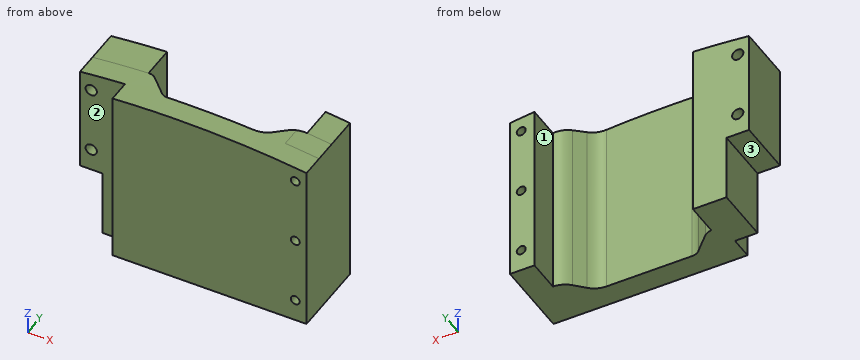
Autodesk Inventor part; units mm, degrees
ref_plane "YZ Plane" through (0, 0, 0) normal (1, 0, 0) x (0, 1, 0)
ref_plane "XZ Plane" through (0, 0, 0) normal (0, 1, 0) x (-1, 0, 0)
ref_plane "XY Plane" through (0, 0, 0) normal (0, 0, 1) x (1, 0, 0)
sketch "Sketch1" plane through (0, 0, 0) normal (0, 0, 1) x (1, 0, 0)
  line L0 (-43.6429, 8.5714) -> (-63.6429, 8.5714)
  line L1 (-63.6429, 8.5714) -> (-63.6429, 18.5714)
  line L2 (-63.6429, 18.5714) -> (-28.6429, 18.5714)
  line L3 (-28.6429, 18.5714) -> (-28.6429, 8.5714)
  line L4 (-28.6429, 8.5714) -> (42.5571, 8.5714)
  line L5 (42.5571, 8.5714) -> (42.5571, -1.4286)
  line L6 (42.5571, -1.4286) -> (-43.6429, -1.4286)
  line L7 (-43.6429, -1.4286) -> (-43.6429, 8.5714)
  point P0 (0, 0)
  dimension "d0" = 10
  dimension "d1" = 10
  dimension "d2" = 20
  dimension "d3" = 86.2
  dimension "d4" = 15
extrude "Extrusion1" add sketch "Sketch1" along normal blind 80
chamfer "Chamfer1" distance 8 angle 45 1 edges at (-28.6429, 18.5714, 40)
fillet "Fillet1" radius 5 2 edges at (-36.6429, 18.5714, 40) (-28.6429, 8.5714, 40)
sketch "Sketch2" plane through (-63.6429, 18.5714, 80) normal (0, 1, 0) x (1, 0, 0)
  circle A0 centre (5, 10) radius 2.5
  circle A1 centre (5, 40) radius 2.5
  line L0 (24.9289, 0) -> (0, 0)
  line L1 (0, 80) -> (0, 0)
  line L2 (0, 80) -> (20, 80)
  line L3 (20, 80) -> (20, 0)
  line L4 (0, 80) -> (10, 80)
  line L5 (10, 80) -> (10, 50)
  line L6 (10, 50) -> (0, 50)
  line L7 (0, 50) -> (0, 80)
  point P0 (63.6429, 80)
  point P1 (20, 50)
  point P2 (0, 50)
  point P3 (10, 80)
  dimension "d11" = 10
  dimension "d12" = 40
  dimension "d13" = 5
  dimension "d14" = 5
  dimension "d15" = 5
  dimension "d16" = 5
  dimension "d31" = 10
extrude "Extrusion2" cut sketch "Sketch2" against normal blind 10 contours A0 | A1 | L1 L2 L5 L6
sketch "Sketch3" plane through (42.5571, 8.5714, 80) normal (0, 1, 0) x (1, 0, 0)
  circle A0 centre (-5, 10) radius 2
  circle A1 centre (-5, 40) radius 2
  circle A2 centre (-5, 70) radius 2
  line L0 (0, 80) -> (0, 0)
  line L1 (0, 80) -> (-67.2, 80)
  line L2 (0, 0) -> (-67.2, 0)
  point P0 (-42.5571, 80)
  dimension "d20" = 4
  dimension "d21" = 4
  dimension "d22" = 4
  dimension "d23" = 5
  dimension "d24" = 5
  dimension "d25" = 5
  dimension "d26" = 10
  dimension "d27" = 40
  dimension "d28" = 10
extrude "Extrusion3" cut sketch "Sketch3" against normal blind 10
sketch "Sketch4" plane through (42.5571, 8.5714, 80) normal (0, 1, 0) x (1, 0, 0)
  arc A0 (-125.8221, 5.2659) -> (2.953, 4.275) centre (-58.1, 438.1) ccw
  line L0 (0, 0) -> (-67.2, 0)
  line L1 (0, 80) -> (0, 0)
  line L2 (2.953, 4.275) -> (3.8116, -7.869)
  line L3 (3.8116, -7.869) -> (-122.3226, -7.869)
  line L4 (-122.3226, -7.869) -> (-125.8221, 5.2659)
  point P0 (-42.5571, 80)
  point P1 (0, 3.8696)
  point P2 (-58.1, 0)
  point P3 (-0.5169, 0)
  dimension "d32" = 876.2
  dimension "d33" = 0
  dimension "d34" = 58.1
extrude "Extrusion4" cut sketch "Sketch4" along normal through all both and the other way through all
sketch "Sketch5" plane through (-24.6429, 8.5714, 0) normal (0, 1, 0) x (1, 0, 0)
  circle A0 centre (62.2, -70) radius 2
  circle A1 centre (62.2, -70) radius 2
  circle A2 centre (62.2, -40) radius 2
  circle A3 centre (62.2, -40) radius 2
  circle A4 centre (62.2, -10) radius 2
  circle A5 centre (62.2, -10) radius 2
  line L0 (67.2, 0) -> (67.2, -80)
  line L1 (67.2, -76.1304) -> (67.2, 0)
  line L2 (67.2, 0) -> (52.2, 0)
  line L3 (67.2, 0) -> (0, 0)
  line L4 (52.2, 0) -> (52.2, -77.8748)
  arc A6 (-19, -79.0979) -> (67.2, -76.1304) centre (9.1, 358.1) ccw
  arc A7 (-55.9, -73.5326) -> (94.1, -73.5326) centre (19.1, 358.0999) ccw
  arc A8 (-55.9, -73.5326) -> (94.1, -73.5326) centre (19.1, 358.0999) ccw
  arc A9 (-55.9, -73.5326) -> (94.1, -73.5326) centre (19.1, 358.0999) ccw
  circle A10 centre (-30.9, 438.0999) radius 2
  circle A11 centre (-30.9, 308.0999) radius 2
  circle A12 centre (69.1, 278.0999) radius 2
  circle A13 centre (69.1, 308.0999) radius 2
  circle A14 centre (69.1, 468.0999) radius 2
  circle A15 centre (-30.9, 468.0999) radius 2
  circle A16 centre (69.1, 408.0999) radius 2
  circle A17 centre (-30.9, 248.0999) radius 2
  circle A18 centre (69.1, 248.0999) radius 2
  circle A19 centre (-30.9, 278.0999) radius 2
  circle A20 centre (-30.9, 408.0999) radius 2
  circle A21 centre (69.1, 438.0999) radius 2
  circle A22 centre (-24, 756.1997) radius 2
  circle A23 centre (62.2, -10) radius 2
  circle A24 centre (62.2, -70) radius 2
  circle A25 centre (-34, -40) radius 2.5
  circle A26 centre (-24, 726.1997) radius 2
  circle A27 centre (-24, 786.1997) radius 2
  circle A28 centre (62.2, -40) radius 2
  circle A29 centre (-34, -70) radius 2.5
  circle A30 centre (72.2, 756.1997) radius 2.5
  circle A31 centre (72.2, 786.1997) radius 2.5
  circle A32 centre (-0.9, 338.0999) radius 2.5
  circle A33 centre (39.1, 338.0999) radius 2.5
  circle A34 centre (-0.9, 378.0999) radius 2.5
  circle A35 centre (39.1, 378.0999) radius 2.5
  circle A36 centre (19.1, 358.0999) radius 7.5
  arc A37 (-55.9, -73.5326) -> (94.1, -73.5326) centre (19.1, 358.0999) ccw
  line L5 (94.1, -73.5326) -> (94.1, 789.7324)
  arc A38 (94.1, 789.7324) -> (-55.9, 789.7324) centre (19.1, 358.0999) ccw
  line L6 (-55.9, 789.7324) -> (-55.9, -73.5326)
  circle A39 centre (69.1, 158.0999) radius 2
  circle A40 centre (-30.9, 38.0999) radius 2
  circle A41 centre (69.1, 558.0999) radius 2
  circle A42 centre (69.1, 518.0999) radius 2
  circle A43 centre (-30.9, 638.0999) radius 2
  circle A44 centre (69.1, 638.0999) radius 2
  circle A45 centre (-30.9, 598.0999) radius 2
  circle A46 centre (69.1, 118.0999) radius 2
  circle A47 centre (-30.9, 118.0999) radius 2
  circle A48 centre (69.1, 78.0999) radius 2
  circle A49 centre (-30.9, 198.0999) radius 2
  circle A50 centre (69.1, 198.0999) radius 2
  circle A51 centre (-30.9, 678.0999) radius 2
  circle A52 centre (-30.9, 558.0999) radius 2
  circle A53 centre (69.1, 678.0999) radius 2
  circle A54 centre (-30.9, 518.0999) radius 2
  circle A55 centre (69.1, 598.0999) radius 2
  circle A56 centre (69.1, 38.0999) radius 2
  circle A57 centre (-30.9, 158.0999) radius 2
  circle A58 centre (-30.9, 78.0999) radius 2
  circle A59 centre (29.9074, 423.6249) radius 2
  circle A60 centre (-0.0926, 473.6249) radius 2
  circle A61 centre (-0.0926, 423.6249) radius 2
  circle A62 centre (29.9074, 473.6249) radius 2
  point P0 (24.6429, 0)
  point P1 (67.0008, -76.157)
  dimension "d37" = 15
extrude "Extrusion5" add sketch "Sketch5" along normal blind 10 contours L0 A6 L4 L2
chamfer "Chamfer2" distance 10 angle 45 1 edges at (27.5571, 8.5714, 38.9374)
fillet "Fillet2" radius 10 3 edges at (17.5572, 8.5714, 39.3739) (27.5571, 18.5713, 38.9374) (27.5571, 18.5714, 38.9374)
sketch "Sketch6" plane through (-24.6429, 18.5714, 0) normal (0, 1, 0) x (1, 0, 0)
  circle A0 centre (62.2, -70) radius 2
  circle A1 centre (62.2, -40) radius 2
  circle A2 centre (62.2, -10) radius 2
  line L0 (56.3421, -77.4454) -> (56.3421, 0)
  arc A3 (56.3421, -77.4454) -> (67.2, -76.1304) centre (9.1, 358.1) ccw
  line L1 (67.2, -76.1304) -> (67.2, 0)
  line L2 (67.2, 0) -> (56.3421, 0)
  circle A4 centre (-34, -70) radius 2.5
  circle A5 centre (-34, -40) radius 2.5
  arc A6 (-39, -77.3515) -> (-14.0711, -79.3868) centre (9.1, 358.1) ccw
  line L3 (-14.0711, 0) -> (-14.0711, -79.3868)
  line L4 (-14.0711, 0) -> (-29, 0)
  line L5 (-29, 0) -> (-29, -30)
  line L6 (-29, -30) -> (-39, -30)
  line L7 (-39, -30) -> (-39, -77.3515)
  point P0 (24.6429, 0)
extrude "Extrusion6" add sketch "Sketch6" along normal blind 14.8
properties part number "ReleaseMec2.0TopPlate"
Geometry check sheet. Reference: the model listing, model coordinates, mm. Face numbers are marked on the shaded views. A direction names the side the tool comes from. Coordinates: 2 decimals unless noted, no trailing zeros. Order: outer loops, then holes, each group sorted by start corner. A loop starts at its lowest first (then second) coordinate and runs counter-clockwise, first axis right, second up. Notation, with made-up numbers: (50, 52.5) - (106, 52.5) arc R16 ccw to (106, 58.5) - close; hole circle Ø2 at (65.5, 24.5). An arc over 180 degrees is marked (long way). Use one line per item in the form item = value.
1. Section check C-C (z = 10). Record the boundary of the cut face in (x, y), then the cut area to 3 significant figures.
Here are the results:
outline = (-53.64, 8.57) - (-43.64, 8.57) - (-43.64, -1.43) - (35.56, -1.43) - (35.56, 33.37) - (31.7, 33.37) - (31.7, 18.57) arc R10 ccw to (24.63, 15.64) - (20.49, 11.5) arc R10 cw to (13.41, 8.57) - (-24.64, 8.57) arc R5 cw to (-28.64, 10.57) - (-35.18, 17.11) arc R5 ccw to (-38.71, 18.57) - (-38.71, 33.37) - (-53.64, 33.37) - close; (39.56, -1.43) - (42.56, -1.43) - (42.56, 33.37) - (39.56, 33.37) - close
area = 1,520 mm²
2. Scan lines: line 1 (X direction, y = 24.5, z = 10); line 2 (X direction, y = 23.25, z = 40); line 3 (X direction, y = 6.5, z = 40). Record each from-to range of solid material in increasing order.
Here are the results:
line_1 = -53.64 to -38.71, 31.7 to 35.56, 39.56 to 42.56
line_2 = -63.64 to -61.14, -56.14 to -38.71, 31.7 to 35.56, 39.56 to 42.56
line_3 = -43.64 to 35.56, 39.56 to 42.56
3. Access from +Z, -Z, +X, -X, +Y, -Y to the whole of each face (thin tool, end or side, straight path). Record for the marked faces 1, 2 and 3.
Here are the results:
face_1 = +Z, -Z, +Y
face_2 = +Z, -Z, -X, -Y
face_3 = -Z, -X, +Y, -Y
4. Section check A-A (y = 28.5). Record the boundary of the cut face in (x, z), then the cut area to 3 significant figures.
Here are the results:
outline = (-63.64, 30) - (-53.64, 30) - (-53.64, 0) - (-38.71, 0) - (-38.71, 79.39) arc R438.07 ccw to (-63.64, 77.35) - close; (31.7, 0) - (42.56, 0) - (42.56, 76.13) arc R438.38 ccw to (31.7, 77.45) - close; hole circle Ø5 at (-58.64, 40); hole circle Ø5 at (-58.64, 70); hole circle Ø4 at (37.56, 10); hole circle Ø4 at (37.56, 40); hole circle Ø4 at (37.56, 70)
area = 2,410 mm²
5. Section check B-B (z = 40). Record the boundary of the cut face in (x, y), then the cut area to 3 significant figures.
Here are the results:
outline = (-63.64, 8.57) - (-61.14, 8.57) - (-61.14, 33.37) - (-63.64, 33.37) - close; (-56.14, 8.57) - (-43.64, 8.57) - (-43.64, -1.43) - (35.56, -1.43) - (35.56, 33.37) - (31.7, 33.37) - (31.7, 18.57) arc R10 ccw to (24.63, 15.64) - (20.49, 11.5) arc R10 cw to (13.41, 8.57) - (-24.64, 8.57) arc R5 cw to (-28.64, 10.57) - (-35.18, 17.11) arc R5 ccw to (-38.71, 18.57) - (-38.71, 33.37) - (-56.14, 33.37) - close; (39.56, -1.43) - (42.56, -1.43) - (42.56, 33.37) - (39.56, 33.37) - close
area = 1,650 mm²
6. Gauge pin test, flat ends, axial feed: pin 1 (2.5 mm diameter, centred on x = 37.56, z = 10, fed in from -Y); pin 2 (1 mm diameter, centred on x = 23.5, z = 28.5, fed in from +Y); pin 3 (12.5 mm diameter, centred on y = 22, z = 16, fed in from -X); pin 4 (5 mm diameter, centred on x = 26.5, z = 62.5, fed in from +Y). Record the tip position at first contact, or that the pin passes through.
Here are the results:
pin_1 = through
pin_2 = 15.01
pin_3 = -53.64
pin_4 = 18.2
7. Section check D-D (z = 49). Record the boundary of the cut face in (x, y).
Here are the results:
outline = (-63.64, 8.57) - (-43.64, 8.57) - (-43.64, -1.43) - (42.56, -1.43) - (42.56, 33.37) - (31.7, 33.37) - (31.7, 18.57) arc R10 ccw to (24.63, 15.64) - (20.49, 11.5) arc R10 cw to (13.41, 8.57) - (-24.64, 8.57) arc R5 cw to (-28.64, 10.57) - (-35.18, 17.11) arc R5 ccw to (-38.71, 18.57) - (-38.71, 33.37) - (-63.64, 33.37) - close
